Read the model definition and answer for the solid it produces. Units are mm, in the model's axes. Coordinates: 2 decimals unless noted, no trailing zeros. Write each loop counter-clockwise with the first axis right and the second up, starting at its lowest first coordinate (ties: lowest second). Pieces come first, ordered by that corner, then holes. Notation, with made-up numbers: (77, 54.25) -> (90, 54.25) arc R24 ccw to (90, 66.25) -> close; hole circle Ø9 at (27, -12.5). An arc over 180 degrees is marked (long way). Use CSV: the item, a comma, the result in double quotes. Start each with the question number.
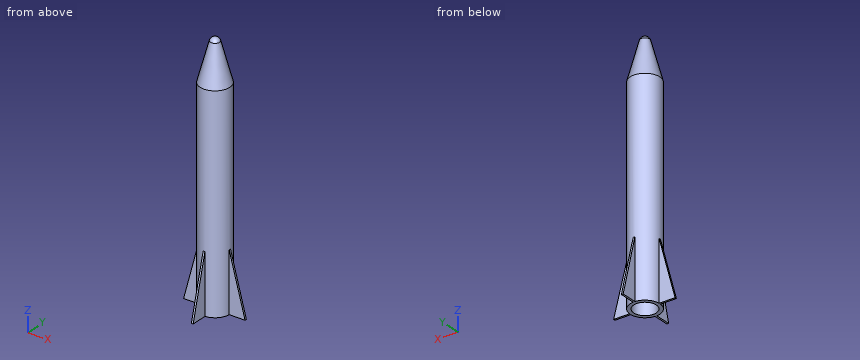
from build123d import *

# Parameters (mm, degrees)
BOSS_EXTRUDE4_REACH      = 217.236
BOSS_EXTRUDE4_END_RADIUS = 12.5
CUT_EXTRUDE1_REACH       = 214.99
CIRPATTERN9_COUNT        = 4


with BuildPart() as part:
    # Sketch1 → Revolve1 (revolve)
    with BuildSketch(Plane.YZ, mode=Mode.PRIVATE) as revolve1_sk:
        with BuildLine():
            Line((-9.5, 0), (-12.5, 0))
            Line((-12.5, 0), (-12.5, 175))
            Line((-12.5, 175), (-3.929753934, 206.98459375))
            ThreePointArc((-3.929753934, 206.98459375), (-2.476673214, 209.15928273), (0, 210))
            Line((0, 210), (0, 206.98459375))
            ThreePointArc((0, 206.98459375), (-0.867879193, 206.03204615), (-1.394318866, 204.855856328))
            Line((-1.394318866, 204.855856328), (-9.5, 174.605042507))
            Line((-9.5, 174.605042507), (-9.5, 80.5))
            Line((-9.5, 80.5), (0, 80.5))
            Line((0, 80.5), (0, 79.5))
            Line((0, 79.5), (-9.5, 70))
            Line((-9.5, 70), (-9.5, 0))
        make_face()
    revolve(revolve1_sk.sketch.rotate(Axis((0, 0, 0), (0, 0, 1)), 270), axis=Axis((0, 0, 0), (0, 0, 1)))

    # Boss-Extrude4: up to this cylinder (the profile starts outside it)
    boss_extrude4_end = Plane(origin=(0, 0, 25), z_dir=(0, 0, -1)) * Cylinder(BOSS_EXTRUDE4_END_RADIUS, 460.472, mode=Mode.PRIVATE)
    # Sketch5 → Boss-Extrude4 (add, up to the surface)
    with BuildSketch(Plane.YZ.offset(33), mode=Mode.PRIVATE) as boss_extrude4_sk1:
        Polygon((0, 0), (-0.75, 0), (-0.75, 50), (0.75, 50), (0.75, 0), align=None)
    boss_extrude4_tool1 = extrude(boss_extrude4_sk1.sketch, amount=-BOSS_EXTRUDE4_REACH, mode=Mode.PRIVATE) - boss_extrude4_end
    boss_extrude4 = boss_extrude4_tool1.solids().sort_by_distance((33, 0, 25))[0]
    add(boss_extrude4)

    # Sketch6 → Cut-Extrude1 (cut, up to next)
    with BuildSketch(Plane(origin=(0, 0.75, 0), x_dir=(-1, 0, 0), z_dir=(0, 1, 0)), mode=Mode.PRIVATE) as cut_extrude1_sk1:
        Polygon((-12.477479713, 50), (-25.874939335, 0), (-33, 0), (-33, 50), align=None)
    cut_extrude1_tool1 = extrude(cut_extrude1_sk1.sketch, amount=-CUT_EXTRUDE1_REACH, mode=Mode.PRIVATE) & part.part
    cut_extrude1 = cut_extrude1_tool1.solids().sort_by_distance((25.547093, 0.75, 29.038165))[0]
    add(cut_extrude1, mode=Mode.SUBTRACT)

    # CirPattern9: Boss-Extrude4, Cut-Extrude1 ×4 about axis
    cirpattern9_axis = Axis((0, 0, 0), (0, 0, 1))
    add([boss_extrude4.rotate(cirpattern9_axis, i * 360 / CIRPATTERN9_COUNT) for i in range(1, CIRPATTERN9_COUNT)])
    add([cut_extrude1.rotate(cirpattern9_axis, i * 360 / CIRPATTERN9_COUNT) for i in range(1, CIRPATTERN9_COUNT)], mode=Mode.SUBTRACT)


solid = part.part
1) Section B-B, the plane x = -19 is taken. Give the vertices of the cut face in (y, z), plus the area to 3 significant figures.
2) Find the intervals of material crossed by line 1 along Y through (x, z) = (0, 56); line 2 along X through (y, z) = (-7, 90); line 3 along X through (y, z) = (7.5, 178.5), in increasing order.
3) Section A-A, the plane z = 160 is taken. Give the vertices of the cut face in (x, y).
4) Section C-C, the plane y = -16 is taken. Give the vertices of the cut face in (x, z), plus the area to 3 significant figures.
5) Each of these flat-tipped pins is pushed along its axis until it touches: pin 1 (14.5 mm diameter, centred on y = 17, z = 30.5, fed in from -X); pin 2 (10 mm diameter, centred on x = -2, z = 47, fed in from -Y); pin 3 (1.5 mm diameter, centred on x = -1, z = 170, fed in from +Y); pin 4 (4 mm diameter, centred on x = 21.5, z = 26.5, fed in from +Y). Where does it stop, or does it pass through?
The answers:
1,outline,"(-0.75, 0) -> (0.75, 0) -> (0.75, 25.66) -> (-0.75, 25.66) -> close"
1,area,"38.5 mm^2"
2,line 1,"y = -12.5 to -9.5, 9.5 to 12.5"
2,line 2,"x = -10.36 to -6.42, 6.42 to 10.36"
2,line 3,"x = -8.8 to -3.91, 3.91 to 8.8"
3,outline,"circle Ø25 at (0, 0); hole circle Ø19 at (0, 0)"
4,outline,"(-0.75, 0) -> (0.75, 0) -> (0.75, 36.85) -> (-0.75, 36.85) -> close"
4,area,"55.3 mm^2"
5,pin 1,"stops at x = -7.82"
5,pin 2,"stops at y = -14.58"
5,pin 3,"stops at y = 12.5"
5,pin 4,"passes through"
